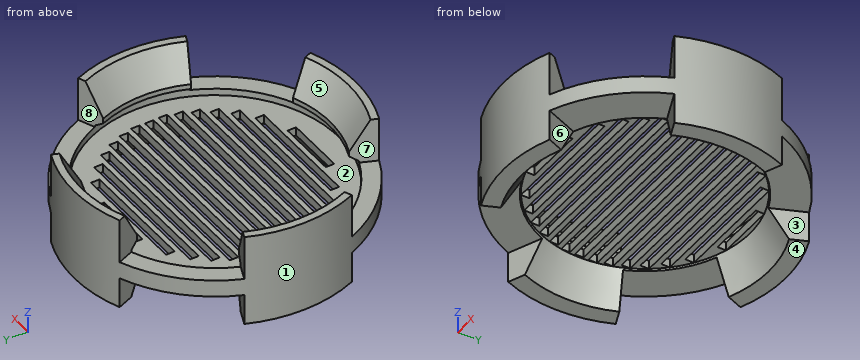
```python
from build123d import *

# Parameters (mm, degrees)
F3_DEPTH      = 9
F4_W          = 60
F4_H          = 2.5
F4_W_2        = 60.1203209974
F4_W_3        = 58.1588600028
F4_W_4        = 54.9768405497
F4_W_5        = 50.3433510687
F4_W_6        = 43.8001483654
F4_W_7        = 17.3911758323
F4_W_8        = 34.2702932119
F5_DEPTH      = 2.5
F5_DEPTH_BACK = 25
F7_DEPTH      = 13


with BuildPart() as f1:
    # F0 (on Front) → F1 (revolve)
    with BuildSketch(Plane.XZ):
        Polygon((-41, 0), (-36, 0), (-30.5151724427, 9.5), (0, 9.5), (0, 12), (-36, 12), (-36, 14.5), (-33.5, 16.25), (-33.5, 17.75), (-38.84048999, 27), (-41, 27), align=None)
    revolve(axis=Axis((0, 0, 37.0227386814), (0, 0, 1)))

    # F2 (on face) → F3 (cut)
    with BuildSketch(Plane(origin=(0, 0, 0), x_dir=(1, 0, 0), z_dir=(0, 0, -1))):
        with BuildLine():
            Line((15.690020727, 37.879060833), (0, 0))
            Line((0, 0), (37.879060833, 15.690020727))
            ThreePointArc((37.879060833, 15.690020727), (28.9913780286, 28.9913780286), (15.690020727, 37.879060833))
        make_face()
        with BuildLine():
            Line((-37.879060833, 15.690020727), (0, 0))
            Line((0, 0), (-15.690020727, 37.879060833))
            ThreePointArc((-15.690020727, 37.879060833), (-28.9913780286, 28.9913780286), (-37.879060833, 15.690020727))
        make_face()
        with BuildLine():
            Line((-15.690020727, -37.879060833), (0, 0))
            Line((0, 0), (-37.879060833, -15.690020727))
            ThreePointArc((-37.879060833, -15.690020727), (-28.9913780286, -28.9913780286), (-15.690020727, -37.879060833))
        make_face()
        with BuildLine():
            Line((37.879060833, -15.690020727), (0, 0))
            Line((0, 0), (15.690020727, -37.879060833))
            ThreePointArc((15.690020727, -37.879060833), (28.9913780286, -28.9913780286), (37.879060833, -15.690020727))
        make_face()
    extrude(amount=-F3_DEPTH, mode=Mode.SUBTRACT)

    # F4 (on face) → F5 (cut, two sides)
    with BuildSketch(Plane(origin=(0, 0, 9.5), x_dir=(1, 0, 0), z_dir=(0, 0, -1))) as f5_sk:
        Rectangle(F4_W, F4_H)
        with Locations((0, -4)):
            Rectangle(F4_W_2, F4_H)
        with Locations((0, -8)):
            Rectangle(F4_W_3, F4_H)
        with Locations((0, -12)):
            Rectangle(F4_W_4, F4_H)
        with Locations((0, -16)):
            Rectangle(F4_W_5, F4_H)
        with Locations((0, -20)):
            Rectangle(F4_W_6, F4_H)
        with Locations((0, -28)):
            Rectangle(F4_W_7, F4_H)
        with Locations((0, -24)):
            Rectangle(F4_W_8, F4_H)
        with Locations((0, 24)):
            Rectangle(F4_W_8, F4_H)
        with Locations((0, 4)):
            Rectangle(F4_W_2, F4_H)
        with Locations((0, 16)):
            Rectangle(F4_W_5, F4_H)
        with Locations((0, 12)):
            Rectangle(F4_W_4, F4_H)
        with Locations((0, 28)):
            Rectangle(F4_W_7, F4_H)
        with Locations((0, 20)):
            Rectangle(F4_W_6, F4_H)
        with Locations((0, 8)):
            Rectangle(F4_W_3, F4_H)
    extrude(amount=-F5_DEPTH, mode=Mode.SUBTRACT)
    extrude(f5_sk.sketch, amount=F5_DEPTH_BACK, mode=Mode.SUBTRACT)

    # F6 (on face) → F7 (cut)
    with BuildSketch(Plane.XY.offset(27)):
        with BuildLine():
            Line((-15.690020727, -37.879060833), (0, 0))
            Line((0, 0), (-37.879060833, -15.690020727))
            ThreePointArc((-37.879060833, -15.690020727), (-28.9913780286, -28.9913780286), (-15.690020727, -37.879060833))
        make_face()
        with BuildLine():
            Line((37.879060833, -15.690020727), (0, 0))
            Line((0, 0), (15.690020727, -37.879060833))
            ThreePointArc((15.690020727, -37.879060833), (28.9913780286, -28.9913780286), (37.879060833, -15.690020727))
        make_face()
        with BuildLine():
            Line((15.690020727, 37.879060833), (0, 0))
            Line((0, 0), (37.879060833, 15.690020727))
            ThreePointArc((37.879060833, 15.690020727), (28.9913780286, 28.9913780286), (15.690020727, 37.879060833))
        make_face()
        with BuildLine():
            Line((-37.879060833, 15.690020727), (0, 0))
            Line((0, 0), (-15.690020727, 37.879060833))
            ThreePointArc((-15.690020727, 37.879060833), (-28.9913780286, 28.9913780286), (-37.879060833, 15.690020727))
        make_face()
    extrude(amount=-F7_DEPTH, mode=Mode.SUBTRACT)


solid = f1.part
```
Source: CAD feature listing. Evaluate the final solid. Frame: model axes, mm. Face numbers are marked on the shaded views. A direction names the side the tool comes from. Coordinates: 2 decimals unless noted, no trailing zeros. Write each loop counter-clockwise with the first axis right and the second up, starting at its lowest first coordinate (ties: lowest second). Pieces come first, ordered by that corner, then holes. Notation, with made-up numbers: M -7,63.25 L 28,63.25 A11 cw 28,82.25 Z; hole C 4.25,84 d2. An arc over 180 degrees is marked long. Answer as a JSON object with one key per item and string values.
1. Ray query, L1, parallel to Y at x = 0, z = 13.6; L2, parallel to X at y = 10, z = 6.75. Return the intervals inside material, ascending.
Evaluation:
{"L1": "-41 to -36, 36 to 41", "L2": "-39.76 to -30.51, 30.51 to 39.76"}
2. Cut plane B-B on z = 18.75. Output: boundary loops of the cut face in (x, y), plus the area to 3 significant figures.
Evaluation:
{"outline": "M -37.88,-15.69 L -31.48,-13.04 A34.08 cw -31.48,13.04 L -37.88,15.69 A41 ccw Z; M -15.69,-37.88 A41 ccw 15.69,-37.88 L 13.04,-31.48 A34.08 cw -13.04,-31.48 Z; M -15.69,37.88 L -13.04,31.48 A34.08 cw 13.04,31.48 L 15.69,37.88 A41 ccw Z; M 31.48,-13.04 L 37.88,-15.69 A41 ccw 37.88,15.69 L 31.48,13.04 A34.08 cw Z", "area": "816 mm^2"}
3. Draft query along X for the marked faces 1, 2, 3 and 4. Return one class per face: released by +X, released by -X, zero draft, split by the parting line, or undercut.
Evaluation:
{"face 1": "split by the parting line", "face 2": "undercut", "face 3": "released by +X", "face 4": "zero draft"}
4. Cut plane C-C on x = 0. State how many separate pieces and enclosed holes the cut face has, plus the area to 3 significant figures.
Evaluation:
{"separate pieces": "16", "enclosed holes": "0", "area": "417 mm^2"}
5. Cut plane A-A on y = 0. Output: boundary loops of the cut face in (x, z), plus the area to 3 significant figures.
Evaluation:
{"outline": "M -41,0 L -36,0 L -30.52,9.5 L -30,9.5 L -30,12 L -36,12 L -36,14.5 L -33.5,16.25 L -33.5,17.75 L -38.84,27 L -41,27 Z; M 30,9.5 L 30.52,9.5 L 36,0 L 41,0 L 41,27 L 38.84,27 L 33.5,17.75 L 33.5,16.25 L 36,14.5 L 36,12 L 30,12 Z", "area": "361 mm^2"}
6. Access query for the marked faces 5, 6, 7 and 8. Directions: +Z, -Z, +X, -X, +Y, -Y. A direction counts if a zero-diameter tool reaches every point of the face in a straight line with its end or side. Return the directions, or none.
Evaluation:
{"face 5": "+Z", "face 6": "-Z, +X", "face 7": "+Z, -X", "face 8": "+Z, +Y"}
7. Contact query for flat-ended pins moving along their axis: P1, Ø3, axis at x = 32, y = -24.5, coming from the -Z side; P2, Ø3, axis at x = 9.5, z = 10, coming from the +Y side; P3, Ø0.6, axis at x = 0, y = -29.5, coming from the -Z side. Output: stop coordinate, or through.
Evaluation:
{"P1": "z = 9", "P2": "y = 40.21", "P3": "z = 9.5"}
